Design review of the part shown in the three views and the two pictorial views. Dimensions are in mm from the part's minimum x, y and z. Round coordinates to 2 decimals unless told otherwise and drop trailing zeros. Order: outer loops, then holes, each group sorted by start corner. A loop starts at its lowest first (then second) coordinate and runs counter-clockwise, first axis right, second up.
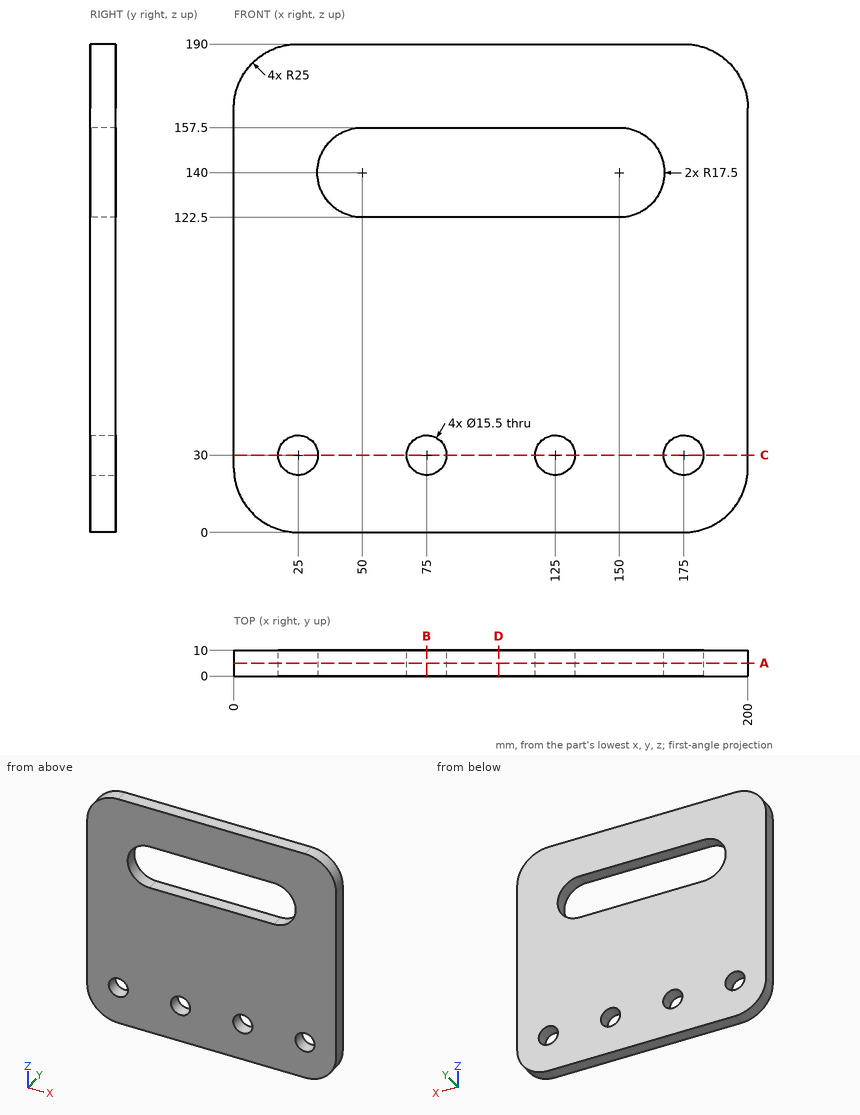
1) Take a section at A-A on y = 5. Give the boundary of the cut face in (x, z).
Results:
outline: (0, 25) arc R25 ccw to (25, 0) - (175, 0) arc R25 ccw to (200, 25) - (200, 165) arc R25 ccw to (175, 190) - (25, 190) arc R25 ccw to (0, 165) - close; hole circle Ø15.5 at (25, 30); hole (50, 122.5) - (150, 122.5) arc R17.5 ccw to (150, 157.5) - (50, 157.5) arc R17.5 ccw to start; hole circle Ø15.5 at (75, 30); hole circle Ø15.5 at (125, 30); hole circle Ø15.5 at (175, 30)
2) Take a section at B-B on x = 75. Give the boundary of the cut face in (y, z).
Results:
outline: (0, 0) - (10, 0) - (10, 22.25) - (0, 22.25) - close; (0, 37.75) - (10, 37.75) - (10, 122.5) - (0, 122.5) - close; (0, 157.5) - (10, 157.5) - (10, 190) - (0, 190) - close
3) Take a section at C-C on z = 30. Give the boundary of the cut face in (x, y).
Results:
outline: (0, 0) - (17.25, 0) - (17.25, 10) - (0, 10) - close; (32.75, 0) - (67.25, 0) - (67.25, 10) - (32.75, 10) - close; (82.75, 0) - (117.25, 0) - (117.25, 10) - (82.75, 10) - close; (132.75, 0) - (167.25, 0) - (167.25, 10) - (132.75, 10) - close; (182.75, 0) - (200, 0) - (200, 10) - (182.75, 10) - close
4) To check wall thickness, follow line 1 along Z through (x, y) = (125, 7.25); line 2 along Z through (x, y) = (150.5, 4); line 3 along Z through (x, y) = (175, 7). State the ranges of each line that lie inside material, in increasing order.
Results:
line 1: z = 0 to 22.25, 37.75 to 122.5, 157.5 to 190
line 2: z = 0 to 122.51, 157.49 to 190
line 3: z = 0 to 22.25, 37.75 to 190
5) Take a section at D-D on x = 103. Give the boundary of the cut face in (y, z), plus the area to 3 significant figures.
Results:
outline: (0, 0) - (10, 0) - (10, 122.5) - (0, 122.5) - close; (0, 157.5) - (10, 157.5) - (10, 190) - (0, 190) - close
area: 1,550 mm2
